The listing builds one solid part. Answer for the finished solid, in the listing's coordinates (mm). A direction names the side the tool comes from. Round coordinates to 2 decimals unless told otherwise and drop trailing zeros. Write each loop counter-clockwise with the first axis right and the second up, starting at its lowest first coordinate (ties: lowest second). Pieces come first, ordered by that corner, then holes. Notation, with made-up numbers: M 64,58 L 76,58 A38 ccw 76,97 Z; hole C -34,21.25 d9. An arc over 180 degrees is marked long. One line per item, written item: value. Start each with the question number.
(1) Section B-B (y = -4.5) is taken. Determine the outline of the cut face in (x, z), plus the area to 3 significant figures.
(2) For faces 5 (the flat face through (0, 0, -2.25)), 6 (the flat face through (0, 25, 0)), determine the directions among +Z, -Z, +X, -X, +Y, -Y from which every point of the face is accessible in a straight line to the end or side of a thin tool.
(3) Given P1, Ø0.8, axis at x = 0, y = -10, coming from the +Z side; P2, Ø1.2, axis at x = 1.5, y = -3.5, coming from the +Z side, each flat-ended and moving along its own axis, determine where each tip first touches the part or whether it passes through.
(4) Section A-A (z = 1.7) is taken. Determine the outline of the cut face in (x, y).
(5) Section C-C (x = 2.5) is taken. Determine the outline of the cut face in (y, z), plus the area to 3 significant figures.
(6) For a pull along Y with two mould halves and no side action, classify faces 1 (the flat face through (0, -26, 0)), 2 (the flat face through (0, 26, 0)), 3 (the flat face through (4, 0, 0)), 4 (the flat face through (-0.5, 0, -1)) as released by +Y, released by -Y, zero draft, split by the parting line, or undercut.
(7) Consider probe 1 along X at (y, z) = (-16, -0.85); probe 2 along Y at (x, z) = (0.25, 2.15); probe 3 along X at (y, z) = (-1, -0.1). Determine where each line is inside the solid, lowest interval first.
Solid Edge part; units mm, degrees
sketch "Sketch1" plane through (0, 0, 0) normal (0, -1, 0) x (1, 0, 0)
  line L0 (4, -2.25) -> (4, 2.25)
  line L1 (4, 2.25) -> (-4, 2.25)
  line L2 (-4, 2.25) -> (-4, -2.25)
  line L3 (-4, -2.25) -> (4, -2.25)
extrude "Protrusion1" add sketch "Sketch1" along normal mid plane 52
sketch "Sketch2" plane through (0, 0, 0) normal (0, -1, 0) x (1, 0, 0)
  line L0 (-3, -1.25) -> (-3, 2.25)
  line L1 (-3, 2.25) -> (3, 2.25)
  line L2 (3, 2.25) -> (3, -1.25)
  line L3 (3, -1.25) -> (0.5, -1.25)
  line L4 (0.5, -1.25) -> (0.5, -0.25)
  line L5 (0.5, -0.25) -> (-0.5, -0.25)
  line L6 (-0.5, -0.25) -> (-0.5, -1.25)
  line L7 (-0.5, -1.25) -> (-3, -1.25)
extrude "Cutout1" cut sketch "Sketch2" along normal mid plane 50
Recorded:
1. outline: M -4,-2.25 L 4,-2.25 L 4,2.25 L 3,2.25 L 3,-1.25 L 0.5,-1.25 L 0.5,-0.25 L -0.5,-0.25 L -0.5,-1.25 L -3,-1.25 L -3,2.25 L -4,2.25 Z
1. area: 16.0 mm2
2. face 5: -Z, +X, -X, +Y, -Y
2. face 6: +Z
3. P1: stops at z = -0.25
3. P2: stops at z = -1.25
4. outline: M -4,-26 L 4,-26 L 4,26 L -4,26 Z; hole M -3,-25 L 3,-25 L 3,25 L -3,25 Z
5. outline: M -26,-2.25 L 26,-2.25 L 26,2.25 L 25,2.25 L 25,-1.25 L -25,-1.25 L -25,2.25 L -26,2.25 Z
5. area: 59.0 mm2
6. face 1: released by -Y
6. face 2: released by +Y
6. face 3: zero draft
6. face 4: undercut
7. probe 1: x = -4 to -3, -0.5 to 0.5, 3 to 4
7. probe 2: y = -26 to -25, 25 to 26
7. probe 3: x = -4 to -3, 3 to 4
